For this review, take the finished solid that the model builds, in its own axes (mm). A direction names the side the tool comes from. Give positions to 0.01 mm unless a question says otherwise; leave off trailing zeros. Order: outer loops, then holes, each group sorted by start corner. A loop starts at its lowest first (then second) coordinate and runs counter-clockwise, first axis right, second up. Notation, with made-up numbers: (-24, -34.75) - (9, -34.75) arc R25 cw to (9, -9.75) - close; hole circle Ø2 at (2.25, 66.25). An arc over 180 degrees is marked (long way). Use a Markdown table: item, result. Add a question column.
1) Wall thickness on L1, parallel to Y at x = 0, z = 13.25; L2, parallel to X at y = -3, z = 6.5; L3, parallel to Y at x = 1.25, z = 9: over which ranges is each line inside the solid? List them lowest first.
2) We need section D-D on z = 3.75. Write out the cut boundary in (x, y), then the cut area to 3 significant figures.
3) Mouldability with a two-part tool opening along X and no side actions: class faces 1 (the face through (-2, 7, 15)), 2 (the face through (-2.086, -9.394, 7.395)), 3 (the face through (2, 0.6, 10.1)) as released by +X, released by -X, zero draft, split by the parting line, or undercut.
4) Clearance check with flat-ended pins moving along their axes: P1, Ø1.5, axis at x = -5.5, z = 3.5, coming from the +Y side; P2, Ø5, axis at x = 4, z = 4, coming from the +Y side; P3, Ø3, axis at y = -3, z = 10, coming from the +X side; P4, Ø7, axis at x = -1.5, y = -1, coming from the +Z side. State where each tip first meets the part, or that it passes through.
5) We need section C-C on z = 9.5. Give the number of separate pieces and of enclosed holes in the cut face, then the cut area to 3 significant figures.
6) Machinability: for faces 4 (the face through (0, 0, 5)), 5 (the face through (2, -2, 15)), which of the approach directions +Z, -Z, +X, -X, +Y, -Y give a long, thin tool a straight path to every point of the face, cutting with its end or side? Answer none if there is none.
7) We need section A-A on y = 0. Write out the cut boundary in (x, z).
```python
from build123d import *

# Parameters (mm, degrees)
F0_R     = 9.623
F1_DEPTH = 15
F2_R     = 2.0875
F3_DEPTH = 10
F2_R_2   = 6.85
F2_R_3   = 4.1625
F4_DEPTH = 10


# Not quite as in the source:
# - a feature names something its author has since deleted; it is built from what else it names


with BuildPart() as f1:
    # F0 (on Top) → F1 (new body)
    with BuildSketch(Plane.XY):
        Circle(F0_R)
    extrude(amount=F1_DEPTH)

    # F2 (on face) → F3 (cut)
    with BuildSketch(Plane.XY.offset(15)):
        Circle(F2_R)
    extrude(amount=-F3_DEPTH, mode=Mode.SUBTRACT)

    # F2 (on face) → F4 (cut)
    with BuildSketch(Plane.XY.offset(15)):
        Circle(F2_R_2)
        Circle(F2_R_3, mode=Mode.SUBTRACT)
    extrude(amount=-F4_DEPTH, mode=Mode.SUBTRACT)


solid = f1.part
```
Checked values:
| question | item | result |
|---|---|---|
| 1 | L1 | -9.62 to -6.85, -4.16 to -2.09, 2.09 to 4.16, 6.85 to 9.62 |
| 1 | L2 | -9.14 to -6.16, -2.89 to 2.89, 6.16 to 9.14 |
| 1 | L3 | -9.54 to -6.73, -3.97 to -1.67, 1.67 to 3.97, 6.73 to 9.54 |
| 2 | outline | circle Ø19.25 at (0, 0) |
| 2 | area | 291 mm² |
| 3 | face 1 | zero draft |
| 3 | face 2 | split by the parting line |
| 3 | face 3 | undercut |
| 4 | P1 | y = 8.37 |
| 4 | P2 | y = 9.51 |
| 4 | P3 | x = 9.51 |
| 4 | P4 | z = 15 |
| 5 | separate pieces | 2 |
| 5 | enclosed holes | 2 |
| 5 | area | 184 mm² |
| 6 | face 4 | +Z |
| 6 | face 5 | +Z, +X, -X, +Y, -Y |
| 7 | outline | (-9.62, 0) - (9.62, 0) - (9.62, 15) - (6.85, 15) - (6.85, 5) - (4.16, 5) - (4.16, 15) - (2.09, 15) - (2.09, 5) - (-2.09, 5) - (-2.09, 15) - (-4.16, 15) - (-4.16, 5) - (-6.85, 5) - (-6.85, 15) - (-9.62, 15) - close |
